Part model, mm, in its own coordinate system. Coordinates: 2 decimals unless noted, no trailing zeros. Loops run counter-clockwise (first coordinate to the right, second up) from the corner with the lowest first, then second, coordinate; pieces in that order, holes last. Notation, with made-up numbers: M -33.75,50 L -26.75,50 A24 ccw -26.75,60 Z; hole C -37.75,-9 d9. An arc over 180 degrees is marked long. Answer as a JSON object with one key per item and string values. Group by question number.
1. Saw through at B-B on z = 0. Write the cut outline in (x, y).
2. Drill centre lines: L1, parallel to X at y = -0.35, z = 0.9; L2, parallel to Z at x = 13.25, y = -1.1; L3, parallel to Y at x = 5.25, z = -1.05. Where is each one in solid material? Low to high.
3. Saw through at A-A on y = 0. Write the cut outline in (x, z).
4. Saw through at C-C on x = 5.75. Write the cut outline in (y, z).
5. Drop flat-ended pins along their axis: pin 1 Ø0.5 at (x, z) = (1, -1) entering from -Y; pin 2 Ø0.5 at (y, z) = (0, 1) entering from -X; pin 3 Ø1.5 at (x, z) = (12, 2) entering from +Y. Give the stop position or say it passes through.
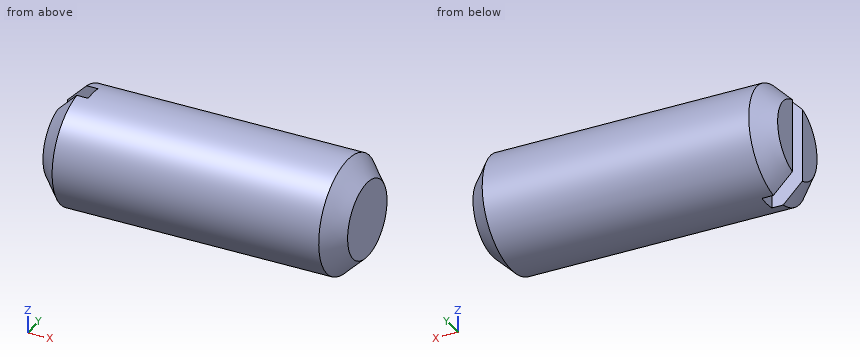
from build123d import *

# Parameters (mm, degrees)
SKETCH_1_R               = 3
EXTRUDE_1_DEPTH          = 16
CUT_EXTRUDE_1_DEPTH      = 17.552945357
CUT_EXTRUDE_1_DEPTH_BACK = 17.552945357
SKETCH_2_W               = 1.6
SKETCH_2_H               = 1
CHAMFER_1_SIZE           = 1


with BuildPart() as part:
    # Эскиз1 → Бобышка-Вытянуть1 (new body)
    with BuildSketch(Plane(origin=(0, 0, 0), x_dir=(0, 0, -1), z_dir=(1, 0, 0))):
        Circle(SKETCH_1_R)
    extrude(amount=EXTRUDE_1_DEPTH)

    # Эскиз2 → Вырез-Вытянуть1 (cut, two sides: drawn at the far end of the back side and taken through both)
    with BuildSketch(Plane.XY.offset(-CUT_EXTRUDE_1_DEPTH_BACK)):
        with Locations((0.8, 0)):
            Rectangle(SKETCH_2_W, SKETCH_2_H)
    extrude(amount=CUT_EXTRUDE_1_DEPTH + CUT_EXTRUDE_1_DEPTH_BACK, mode=Mode.SUBTRACT)

    # Фаска1
    chamfer_1_edges = [part.edges().sort_by_distance(p)[0] for p in [
        (16, 0, 3),
        (0, 3, 0),
        (0, -3, 0),
    ]]
    chamfer(chamfer_1_edges, length=CHAMFER_1_SIZE)


solid = part.part
Outcome:
{
 "1": {"outline": "M 0,-2 L 1,-3 L 15,-3 L 16,-2 L 16,2 L 15,3 L 1,3 L 0,2 L 0,0.5 L 1.6,0.5 L 1.6,-0.5 L 0,-0.5 Z"},
 "2": {"L1": "x = 1.6 to 16", "L2": "z = -2.79 to 2.79", "L3": "y = -2.81 to 2.81"},
 "3": {"outline": "M 1.6,-3 L 15,-3 L 16,-2 L 16,2 L 15,3 L 1.6,3 Z"},
 "4": {"outline": "C 0,0 d6"},
 "5": {"pin 1": "stops at y = -2.9", "pin 2": "stops at x = 1.6", "pin 3": "stops at y = 2.73"}
}
